from build123d import *

# Parameters (mm, degrees)
SKETCH1_W           = 30
SKETCH1_H           = 10
SKETCH1_R           = 1.5
BOSS_EXTRUDE1_DEPTH = 3
SKETCH2_W           = 10
SKETCH2_H           = 80
BOSS_EXTRUDE2_DEPTH = 3


with BuildPart() as part:
    # Sketch1 → Boss-Extrude1 (new body)
    with BuildSketch(Plane(origin=(0, 0, 0), x_dir=(1, 0, 0), z_dir=(0, 1, 0))):
        Rectangle(SKETCH1_W, SKETCH1_H)
        Circle(SKETCH1_R, mode=Mode.SUBTRACT)
    extrude(amount=BOSS_EXTRUDE1_DEPTH)

    # Sketch2 → Boss-Extrude2 (add)
    with BuildSketch(Plane(origin=(0, 0, 0), x_dir=(1, 0, 0), z_dir=(0, 1, 0))):
        with Locations((0, -45)):
            Rectangle(SKETCH2_W, SKETCH2_H)
        with BuildLine():
            Line((-1.5, -8), (-1.5, -78))
            ThreePointArc((-1.5, -78), (0, -79.5), (1.5, -78))
            Line((1.5, -78), (1.5, -8))
            ThreePointArc((1.5, -8), (0, -6.5), (-1.5, -8))
        make_face(mode=Mode.SUBTRACT)
    extrude(amount=BOSS_EXTRUDE2_DEPTH)


solid = part.part
Input: part model. Units: mm. Frame: model coordinates. A direction names the side the tool comes from. Coordinates: 2 decimals unless noted, no trailing zeros. Loops run counter-clockwise (first coordinate to the right, second up) from the corner with the lowest first, then second, coordinate; pieces in that order, holes last.
Q1. Contact query for flat-ended pins moving along their axis: pin 1 (1.8 mm diameter, centred on x = 0, z = 0, fed in from -Y); pin 2 (6 mm diameter, centred on x = 6, z = 13.5, fed in from -Y); pin 3 (1 mm diameter, centred on x = 9.5, y = 1, fed in from +Z); pin 4 (1.5 mm diameter, centred on y = 2, z = 40, fed in from +X). Output: stop coordinate, or through.
Q2. Cut plane D-D (z = 24). Output: boundary loops of the cut face in (x, y).
Q3. Cut plane B-B (z = 0). Output: boundary loops of the cut face in (x, y).
Q4. Draft query along Z for faces 1 (the face through (2, 0, 30)), 2 (the face through (0, 1.5, 79.5)), 3 (the face through (0, 1, -5)), 4 (the face through (-10, 1, 5)). Return one class per face: +Z half, -Z half, draft (parallel to the pull), parting line (faces both ways), or undercut.
Q5. Cut plane A-A (x = 0). Output: boundary loops of the cut face in (y, z).
Q6. Set-up query: faces 5 (the face through (-1.5, 1, 43)), 6 (the face through (-5, 1, 46)), 7 (the face through (15, 1, 0)), 8 (the face through (10, 1, 5)), 9 (the face through (0, 1, 85)). Return all of +Z, -Z, +X, -X, +Y, -Y with unobstructed straight access to the full face (end or side cutting, diameter ignored); none if empty.
Q7. Material intervals for line 1 (Z direction, x = 0, y = 0.75); line 2 (X direction, y = 0.3, z = 62); line 3 (Z direction, x = -1, y = 1), sorted ascending.
Q8. Cut plane C-C (y = 2.5). Output: boundary loops of the cut face in (x, z), then the cut area to 3 significant figures.
Working result:
1. pin 1: passes through
1. pin 2: stops at y = 0
1. pin 3: stops at z = 5
1. pin 4: stops at x = 5
2. outline: (-5, 0) - (-1.5, 0) - (-1.5, 3) - (-5, 3) - close; (1.5, 0) - (5, 0) - (5, 3) - (1.5, 3) - close
3. outline: (-15, 0) - (-1.5, 0) - (-1.5, 3) - (-15, 3) - close; (1.5, 0) - (15, 0) - (15, 3) - (1.5, 3) - close
4. face 1: draft
4. face 2: undercut
4. face 3: -Z half
4. face 4: +Z half
5. outline: (0, -5) - (3, -5) - (3, -1.5) - (0, -1.5) - close; (0, 1.5) - (3, 1.5) - (3, 6.5) - (0, 6.5) - close; (0, 79.5) - (3, 79.5) - (3, 85) - (0, 85) - close
6. face 5: +Y, -Y
6. face 6: +Z, -X, +Y, -Y
6. face 7: +Z, -Z, +X, +Y, -Y
6. face 8: +Z, +X, +Y, -Y
6. face 9: +Z, +X, -X, +Y, -Y
7. line 1: z = -5 to -1.5, 1.5 to 6.5, 79.5 to 85
7. line 2: x = -5 to -1.5, 1.5 to 5
7. line 3: z = -5 to -1.12, 1.12 to 6.88, 79.12 to 85
8. outline: (-15, -5) - (15, -5) - (15, 5) - (5, 5) - (5, 85) - (-5, 85) - (-5, 5) - (-15, 5) - close; hole circle Ø3 at (0, 0); hole (-1.5, 8) arc R1.5 ccw to (1.5, 8) - (1.5, 78) arc R1.5 ccw to (-1.5, 78) - close
8. area: 876 mm2
